```python
from build123d import *

# Parameters (mm, degrees)
SKETCH1_W           = 20
SKETCH1_H           = 20
BOSS_EXTRUDE1_DEPTH = 4
SKETCH2_R           = 3.7
CUT_EXTRUDE1_DEPTH  = 2.6
SKETCH3_R           = 2.1
CUT_EXTRUDE2_DEPTH  = 29.403520909
SKETCH4_W           = 12
SKETCH4_H           = 4
BOSS_EXTRUDE2_DEPTH = 10
SKETCH7_W           = 20
SKETCH7_H           = 4
BOSS_EXTRUDE3_DEPTH = 10
SKETCH8_W           = 8
SKETCH8_H           = 20
BOSS_EXTRUDE4_DEPTH = 5
SKETCH9_W           = 8
SKETCH9_H           = 20
BOSS_EXTRUDE5_DEPTH = 5
SKETCH10_R          = 1.6
CUT_EXTRUDE5_DEPTH  = 41.012498047
FILLET6_R           = 3
FILLET7_R           = 3
FILLET8_R           = 4


with BuildPart() as part:
    # Sketch1 → Boss-Extrude1 (new body)
    with BuildSketch(Plane(origin=(0, 0, 0), x_dir=(0, 0, -1), z_dir=(1, 0, 0))):
        with Locations((-10, -10)):
            Rectangle(SKETCH1_W, SKETCH1_H)
    extrude(amount=BOSS_EXTRUDE1_DEPTH)

    # Sketch2 → Cut-Extrude1 (cut)
    with BuildSketch(Plane(origin=(4, 0, 0), x_dir=(0, 0, -1), z_dir=(1, 0, 0))):
        with Locations((-10, -10)):
            Circle(SKETCH2_R)
    extrude(amount=-CUT_EXTRUDE1_DEPTH, mode=Mode.SUBTRACT)

    # Sketch3 → Cut-Extrude2 (cut, through all)
    with BuildSketch(Plane(origin=(1.4, 0, 0), x_dir=(0, 0, -1), z_dir=(1, 0, 0))):
        with Locations((-10, -10)):
            Circle(SKETCH3_R)
    extrude(amount=-CUT_EXTRUDE2_DEPTH, mode=Mode.SUBTRACT)

    # Sketch4 → Boss-Extrude2 (add)
    with BuildSketch(Plane(origin=(4, 0, 0), x_dir=(0, 0, -1), z_dir=(1, 0, 0))):
        Polygon((-20, 0), (-20, -20), (-16, -20), (-16, -16), (-16, -4), (-16, 0), align=None)
        with Locations((-10, -18)):
            Rectangle(SKETCH4_W, SKETCH4_H)
        Polygon((-4, -16), (-4, -20), (0, -20), (0, -4), (-4, -4), align=None)
        Polygon((0, 0), (-16, 0), (-16, -4), (-4, -4), (0, -4), align=None)
    extrude(amount=BOSS_EXTRUDE2_DEPTH)

    # Sketch7 → Boss-Extrude3 (add)
    with BuildSketch(Plane(origin=(14, 0, 0), x_dir=(0, 0, -1), z_dir=(1, 0, 0))):
        with Locations((-10, -18)):
            Rectangle(SKETCH7_W, SKETCH7_H)
        with Locations((-10, -2)):
            Rectangle(SKETCH7_W, SKETCH7_H)
    extrude(amount=BOSS_EXTRUDE3_DEPTH)

    # Sketch8 → Boss-Extrude4 (add)
    with BuildSketch(Plane(origin=(0, -20, 0), x_dir=(-1, 0, 0), z_dir=(0, -1, 0))):
        with Locations((-20, -10)):
            Rectangle(SKETCH8_W, SKETCH8_H)
    extrude(amount=BOSS_EXTRUDE4_DEPTH)

    # Sketch9 → Boss-Extrude5 (add)
    with BuildSketch(Plane(origin=(0, 0, 0), x_dir=(1, 0, 0), z_dir=(0, 1, 0))):
        with Locations((20, -10)):
            Rectangle(SKETCH9_W, SKETCH9_H)
    extrude(amount=BOSS_EXTRUDE5_DEPTH)

    # Sketch10 → Cut-Extrude5 (cut, through all)
    with BuildSketch(Plane(origin=(0, 0, 0), x_dir=(-1, 0, 0), z_dir=(0, 0, -1))):
        with Locations(Location((-20, 1, 0), (0, 0, 90))):
            Circle(SKETCH10_R)
        with Locations(Location((-20, -21, 0), (0, 0, 90))):
            Circle(SKETCH10_R)
    extrude(amount=-CUT_EXTRUDE5_DEPTH, mode=Mode.SUBTRACT)

    # Fillet6
    fillet6_edges = [part.edges().sort_by_distance(p)[0] for p in [
        (24, -16, 10),
        (24, -4, 10),
        (24, -25, 10),
        (16, -25, 10),
        (24, 5, 10),
        (16, 5, 10),
    ]]
    fillet(fillet6_edges, radius=FILLET6_R)

    # Fillet7
    fillet7_edges = [part.edges().sort_by_distance(p)[0] for p in [
        (9, -4, 16),
        (9, -4, 4),
        (9, -16, 4),
        (9, -16, 16),
        (14, -16, 18),
        (14, -16, 2),
        (14, -4, 2),
        (14, -4, 18),
    ]]
    fillet(fillet7_edges, radius=FILLET7_R)

    # Fillet8
    fillet8_edges = [part.edges().sort_by_distance(p)[0] for p in [
        (16, -20, 10),
        (16, 0, 10),
    ]]
    fillet(fillet8_edges, radius=FILLET8_R)


solid = part.part
```
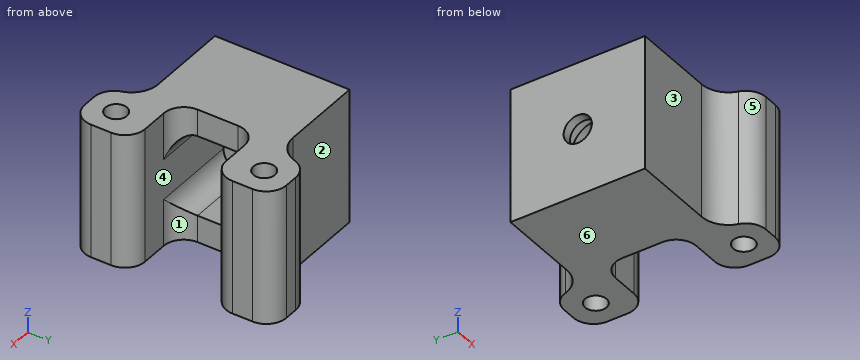
For this review, take the finished solid that the model builds, in its own axes (mm). Face numbers are marked on the shaded views. A direction names the side the tool comes from. Coordinates: 2 decimals unless noted, no trailing zeros. Write each loop counter-clockwise with the first axis right and the second up, starting at its lowest first coordinate (ties: lowest second). Pieces come first, ordered by that corner, then holes.
(1) Add section A-A on x = 20. Give the boundary of the cut face in (y, z), then the cut area to 3 significant figures.
(2) Wall thickness on probe 1 along Y at (x, z) = (19, 12); probe 2 along Y at (x, z) = (3.3, 10); probe 3 along X at (y, z) = (-11, 18.5): over which ranges is each line inside the solid? List them lowest first.
(3) Add section D-D on z = 10. Count the separate pieces of the cut face and the enclosed holes in it, then the cut area to 3 significant figures.
(4) Tool access review of the marked faces 1, 2 and 3: name each direction out of +Z, -Z, +X, -X, +Y, -Y from which nothing blocks a thin tool from reaching the whole face with its end or side.
(5) Add section C-C on x = 8.5. Give the boundary of the cut face in (y, z).
(6) The part is to be moulded in two halves that separate along Y. For the marked faces 4, 5 and 6, say which applies: +Y half, -Y half, draft (parallel to the pull), parting line (faces both ways), or undercut.
(7) For pin 1 Ø10 at (x, y) = (14, -1.5) entering from -Z; pin 2 Ø3.5 at (y, z) = (-12, 10) entering from +X; pin 3 Ø5 at (x, z) = (12, 6) entering from +Y; pin 4 Ø4.5 at (y, z) = (-9, 17) entering from +X, all flat-tipped, find the tip position at first contact; note any pin that passes through.
(8) Add section B-B on y = -10. Give the boundary of the cut face in (x, z).
Answer sheet:
1. outline: (-25, 0) - (-22.6, 0) - (-22.6, 20) - (-25, 20) - close; (-19.4, 0) - (-16, 0) - (-16, 20) - (-19.4, 20) - close; (-4, 0) - (-0.6, 0) - (-0.6, 20) - (-4, 20) - close; (2.6, 0) - (5, 0) - (5, 20) - (2.6, 20) - close
1. area: 232 mm2
2. probe 1: y = -25 to -22.25, -19.75 to -16, -4 to -0.25, 2.25 to 5
2. probe 2: y = -20 to -13.7, -6.3 to 0
2. probe 3: x = 0 to 14
3. separate pieces: 2
3. enclosed holes: 2
3. area: 272 mm2
4. face 1: +Z, -Z, +X
4. face 2: +Z, -Z, -X, +Y
4. face 3: +Z, -Z, -X, -Y
5. outline: (-20, 0) - (0, 0) - (0, 20) - (-20, 20) - close; hole (-16, 7) arc R3 ccw to (-13, 4) - (-7, 4) arc R3 ccw to (-4, 7) - (-4, 13) arc R3 ccw to (-7, 16) - (-13, 16) arc R3 ccw to (-16, 13) - close
6. face 4: undercut
6. face 5: -Y half
6. face 6: draft
7. pin 1: stops at z = 0
7. pin 2: stops at x = 4
7. pin 3: stops at y = 0.66
7. pin 4: stops at x = 14.01
8. outline: (0, 0) - (14, 0) - (14, 4) - (4, 4) - (4, 6.3) - (1.4, 6.3) - (1.4, 7.9) - (0, 7.9) - close; (0, 12.1) - (1.4, 12.1) - (1.4, 13.7) - (4, 13.7) - (4, 16) - (14, 16) - (14, 20) - (0, 20) - close
